Autodesk Inventor part; units mm, degrees
ref_plane "Work Plane1" through (0, 18.542, 0) normal (0, 1, 0) x (1, 0, 0)
ref_plane "YZ Plane" through (0, 0, 0) normal (1, 0, 0) x (0, 1, 0)
ref_plane "XZ Plane" through (0, 0, 0) normal (0, 1, 0) x (-1, 0, 0)
sketch "Sketch1" plane through (0, 0, 0) normal (0, 1, 0) x (-1, 0, 0)
  line L0 (1.27, 0) -> (11.43, 0)
  line L1 (12.7, -1.27) -> (12.7, -21.59)
  line L2 (11.43, -22.86) -> (1.27, -22.86)
  line L3 (0, -21.59) -> (0, -1.27)
  arc A0 (12.7, -1.27) -> (11.43, 0) centre (11.43, -1.27) ccw
  arc A1 (1.27, 0) -> (0, -1.27) centre (1.27, -1.27) ccw
  arc A2 (0, -21.59) -> (1.27, -22.86) centre (1.27, -21.59) ccw
  arc A3 (11.43, -22.86) -> (12.7, -21.59) centre (11.43, -21.59) ccw
  point P0 (0, 0)
  point P1 (12.7, -22.86)
  point P2 (12.7, 0)
  point P3 (0, -22.86)
  dimension "d0" = 12.7
  dimension "d1" = 22.86
  dimension "d2" = 1.27
extrude "Extrusion1" add sketch "Sketch1" along normal blind 22.86
sketch "Sketch2" plane through (0, 22.86, 0) normal (0, 1, 0) x (1, 0, 0)
  line L0 (-12.7, 21.59) -> (-12.7, 1.27)
  line L1 (-11.43, 0) -> (-1.27, 0)
  line L2 (0, 1.27) -> (0, 21.59)
  circle A0 centre (-6.35, 6.35) radius 6.35
  point P0 (0, 0)
extrude "Extrusion2" add sketch "Sketch2" along normal blind 5.08
sketch "Sketch3" plane through (-6.35, 27.94, -6.35) normal (0, 1, 0) x (1, 0, 0)
  circle A0 centre (0, 0) radius 12.065
  point P0 (6.35, -6.35)
  dimension "d9" = 24.13
extrude "Extrusion3" add sketch "Sketch3" along normal blind 4.064
ref_plane "Work Plane1" through (0, 18.542, 0) normal (0, 1, 0) x (1, 0, 0)
sketch "Sketch5" plane through (0, 18.542, 0) normal (0, 1, 0) x (1, 0, 0)
  line L0 (-12.7, 27.432) -> (0, 27.432)
  line L1 (-12.7, 21.59) -> (-12.7, 1.27)
  line L2 (0, 1.27) -> (0, 21.59)
  circle A0 centre (-6.35, 24.13) radius 1.016
  line L3 (0, 11.43) -> (-12.7, 11.43) construction
  line L4 (-12.7, -4.572) -> (0, -4.572)
  circle A1 centre (-6.35, -1.27) radius 1.016
  line L5 (-12.7, -4.572) -> (-12.7, 27.432)
  line L6 (0, 27.432) -> (0, -4.572)
  point P0 (0, 0)
  dimension "d13" = 16.002
  dimension "d14" = 2.032
  dimension "d15" = 25.4
extrude "Extrusion4" add sketch "Sketch5" against normal blind 2.54
sketch "Sketch6" plane through (-11.43, 0, 0) normal (0, 0, 1) x (1, 0, 0)
  line L0 (3.429, 5.334) -> (6.731, 5.334)
  line L1 (6.731, 5.334) -> (6.731, 4.318)
  line L2 (6.731, 4.318) -> (3.429, 4.318)
  line L3 (3.429, 4.318) -> (3.429, 5.334)
  line L4 (0, 0) -> (10.16, 0)
  point P0 (11.43, 0)
  point P1 (5.08, 0)
  point P2 (5.08, 4.318)
  dimension "d18" = 3.302
  dimension "d19" = 1.016
  dimension "d20" = 4.318
extrude "Extrusion5" add sketch "Sketch6" along normal blind 2.54
properties part number "servo (2)"
The model under review builds one solid part; all positions refer to its coordinate system, in mm. A direction names the side the tool comes from. Coordinates: 2 decimals unless noted, no trailing zeros. Write each loop counter-clockwise with the first axis right and the second up, starting at its lowest first coordinate (ties: lowest second). Pieces come first, ordered by that corner, then holes. Notation, with made-up numbers: (54, 31.5) - (81, 31.5) arc R28 ccw to (81, 55.5) - close; hole circle Ø2 at (39, 13). An arc over 180 degrees is marked (long way). Answer as CSV lines item,"result".
(1) Tool access review of faces 4 (the cylindrical face through (-0.382, 20.671, -22.498)), 5 (the flat face through (-8.001, 5, 1)), 6 (the cylindrical face through (-12.338, 7.889, -22.478)), 7 (the cylindrical face through (-12.338, 20.671, -22.478)): name each direction out of +Z, -Z, +X, -X, +Y, -Y from which nothing blocks a thin tool from reaching the whole face with its end or side.
Data:
face 4,"-Z, +X, +Y"
face 5,"+Z, -X, -Y"
face 6,"-Z, -X, -Y"
face 7,"-Z, -X, +Y"
(2) We need section A-A (z = -24.13). Give the boundary of the cut face in (x, y).
Data:
outline,"(-12.7, 16) - (-7.37, 16) - (-7.37, 18.54) - (-12.7, 18.54) - close; (-5.33, 16) - (0, 16) - (0, 18.54) - (-5.33, 18.54) - close"
(3) For line 1 along X through (y, z) = (18.05, -24.13); line 2 along Z through (x, y) = (-6.35, 17.4); line 3 along Y through (x, z) = (-0.5, -1.5), list the stretches that pass through material, from the lowest coordinate up. Write a range as [from, to].
Data:
line 1,"x = [-12.7, -7.37], [-5.33, 0]"
line 2,"z = [-27.43, -25.15], [-23.11, 0.25], [2.29, 4.57]"
line 3,"y = [0, 22.86], [27.94, 32]"
(4) We need section D-D (z = -4). Give the boundary of the cut face in (x, y).
Data:
outline,"(-18.18, 27.94) - (-12.25, 27.94) - (-12.25, 22.86) - (-12.7, 22.86) - (-12.7, 0) - (0, 0) - (0, 22.86) - (-0.45, 22.86) - (-0.45, 27.94) - (5.48, 27.94) - (5.48, 32) - (-18.18, 32) - close"
(5) Clearance check with flat-ended pins moving along their axes: pin 1 Ø3 at (x, y) = (-15.5, 12) entering from -Z; pin 2 Ø0.8 at (x, y) = (-6, 5) entering from +Z; pin 3 Ø8 at (y, z) = (4.5, -14.5) entering from -X; pin 4 Ø3 at (x, y) = (-8.5, 5) entering from -Z. State where each tip first meets the part, or that it passes through.
Data:
pin 1,"passes through"
pin 2,"stops at z = 2.54"
pin 3,"stops at x = -12.7"
pin 4,"stops at z = -22.86"
(6) We need section C-C (z = 1.27). Give the boundary of the cut face in (x, y), plus the area to 3 significant figures.
Data:
outline,"(-15.7, 27.94) - (3, 27.94) - (3, 32) - (-15.7, 32) - close; (-12.7, 16) - (-7.37, 16) - (-7.37, 18.54) - (-12.7, 18.54) - close; (-8, 4.32) - (-4.7, 4.32) - (-4.7, 5.33) - (-8, 5.33) - close; (-5.33, 16) - (0, 16) - (0, 18.54) - (-5.33, 18.54) - close"
area,"106 mm2"
(7) Mouldability with a two-part tool opening along X and no side actions: class faces 1 (the flat face through (0, 12, -12)), 2 (the flat face through (-1, 27.94, -1)), 3 (the cylindrical face through (-7.365, 17.29, 1.225)) as pulls with the +X half, pulls with the -X half, needs draft (parallel to the pull), parting line crosses it, or undercut.
Data:
face 1,"pulls with the +X half"
face 2,"needs draft"
face 3,"undercut"
(8) We need section B-B (y = 11). Give the boundary of the cut face in (x, z).
Data:
outline,"(-12.7, -21.59) arc R1.27 ccw to (-11.43, -22.86) - (-1.27, -22.86) arc R1.27 ccw to (0, -21.59) - (0, -1.27) arc R1.27 ccw to (-1.27, 0) - (-11.43, 0) arc R1.27 ccw to (-12.7, -1.27) - close"
